Verification items for the finished model (mm, model axes). A direction names the side the tool comes from. Give positions to 0.01 mm unless a question says otherwise; leave off trailing zeros. Loops run counter-clockwise (first coordinate to the right, second up) from the corner with the lowest first, then second, coordinate; pieces in that order, holes last. Notation, with made-up numbers: M 50.5,24 L 86.5,24 A7 ccw 86.5,34 Z; hole C 56,4.25 d7. An arc over 180 degrees is marked long. Use a Markdown table: item, result.
from build123d import *

# Parameters (mm, degrees)
SKETCH1_R           = 25
BOSS_EXTRUDE1_DEPTH = 14
SKETCH2_R           = 11
CUT_EXTRUDE1_DEPTH  = 7
SKETCH5_W           = 7.5
SKETCH5_H           = 40
BOSS_EXTRUDE2_DEPTH = 80
FILLET1_R           = 10
SKETCH7_R           = 11
CUT_EXTRUDE3_DEPTH  = 24.5


with BuildPart() as part:
    # Sketch1 → Boss-Extrude1 (new body)
    with BuildSketch(Plane(origin=(0, 0, 0), x_dir=(1, 0, 0), z_dir=(0, 1, 0))):
        with Locations(Location((0, 0, 0), (0, 0, 90))):
            Circle(SKETCH1_R)
    extrude(amount=BOSS_EXTRUDE1_DEPTH)

    # Sketch2 → Cut-Extrude1 (cut)
    with BuildSketch(Plane.XZ):
        with Locations(Location((0, 0, 0), (0, 0, 270))):
            Circle(SKETCH2_R)
    extrude(amount=-CUT_EXTRUDE1_DEPTH, mode=Mode.SUBTRACT)

    # Sketch5 → Boss-Extrude2 (add)
    with BuildSketch(Plane(origin=(0, 14, 0), x_dir=(1, 0, 0), z_dir=(0, 1, 0))):
        with Locations((-8.85, 0)):
            Rectangle(SKETCH5_W, SKETCH5_H)
        with Locations((8.85, 0)):
            Rectangle(SKETCH5_W, SKETCH5_H)
    extrude(amount=BOSS_EXTRUDE2_DEPTH)

    # Fillet1
    fillet1_edges = [part.edges().sort_by_distance(p)[0] for p in [
        (-8.85, 94, 20),
        (-8.85, 94, -20),
        (8.85, 94, 20),
        (8.85, 94, -20),
    ]]
    fillet(fillet1_edges, radius=FILLET1_R)

    # Sketch7 → Cut-Extrude3 (cut)
    with BuildSketch(Plane.ZY.offset(12.6)):
        with Locations((0, 79)):
            Circle(SKETCH7_R)
    extrude(amount=-CUT_EXTRUDE3_DEPTH, mode=Mode.SUBTRACT)


solid = part.part
(1) Draft check along Z on faces 1 (the flat face through (11, 0, -5)), 2 (the cylindrical face through (8.9, 90.99, -17.15)), 3 (the flat face through (0, 7, 0)), 4 (the cylindrical face through (-8.8, 90.99, 17.15)). Enter one of: +Z half, -Z half, draft (parallel to the pull), parting line (faces both ways), or undercut.
Results below:
| item | result |
|---|---|
| face 1 | draft |
| face 2 | -Z half |
| face 3 | undercut |
| face 4 | +Z half |
(2) Material ranges on line 1 (X direction, y = 31.5, z = 17.5); line 2 (Y direction, x = 7.25, z = 0); line 3 (X direction, y = 4, z = 0), recorded low to high.
Results below:
| item | result |
|---|---|
| line 1 | -12.6 to -5.1, 5.1 to 12.6 |
| line 2 | 7 to 68, 90 to 94 |
| line 3 | -25 to -11, 11 to 25 |
(3) Set-up check for faces 5 (the flat face through (-5.1, 53, 0)), 6 (the flat face through (12.6, 53, 0)), 7 (the flat face through (9, 49, 20)), 8 (the cylindrical face through (8.452, 89.906, -1.432)), 9 (the flat face through (-9, 49, -20)): record each of +Z, -Z, +X, -X, +Y, -Y from which the full face is reachable in a straight line by a thin tool's end or side.
Results below:
| item | result |
|---|---|
| face 5 | +Z, -Z, +Y |
| face 6 | +Z, -Z, +X, +Y |
| face 7 | +Z, +X, -X, +Y |
| face 8 | -X |
| face 9 | -Z, +X, -X, +Y |
(4) Cross-section at A-A on y = 79. Record the cut outline in (x, z), then the cut area to 3 significant figures.
Results below:
| item | result |
|---|---|
| outline | M -12.6,-20 L -5.1,-20 L -5.1,-11 L -12.6,-11 Z; M -12.6,11 L -5.1,11 L -5.1,20 L -12.6,20 Z; M 5.1,-20 L 12.6,-20 L 12.6,20 L 5.1,20 L 5.1,11 L 11.9,11 L 11.9,-11 L 5.1,-11 Z |
| area | 285 mm^2 |
(5) Cross-section at C-C on z = 0. Record the cut outline in (x, y), then the cut area to 3 significant figures.
Results below:
| item | result |
|---|---|
| outline | M -25,0 L -11,0 L -11,7 L 11,7 L 11,0 L 25,0 L 25,14 L 12.6,14 L 12.6,94 L 5.1,94 L 5.1,90 L 11.9,90 L 11.9,68 L 5.1,68 L 5.1,14 L -5.1,14 L -5.1,68 L -12.6,68 L -12.6,14 L -25,14 Z; M -12.6,90 L -5.1,90 L -5.1,94 L -12.6,94 Z |
| area | 1,430 mm^2 |
(6) Cross-section at D-D on z = -5. Record the cut outline in (x, y), then the cut area to 3 significant figures.
Results below:
| item | result |
|---|---|
| outline | M -24.49,0 L -9.8,0 L -9.8,7 L 9.8,7 L 9.8,0 L 24.49,0 L 24.49,14 L 12.6,14 L 12.6,94 L 5.1,94 L 5.1,88.8 L 11.9,88.8 L 11.9,69.2 L 5.1,69.2 L 5.1,14 L -5.1,14 L -5.1,69.2 L -12.6,69.2 L -12.6,14 L -24.49,14 Z; M -12.6,88.8 L -5.1,88.8 L -5.1,94 L -12.6,94 Z |
| area | 1,470 mm^2 |
(7) Gauge pin test, flat ends, axial feed: P1, Ø8, axis at x = 10.5, y = 63, coming from the -Z side; P2, Ø1.5, axis at y = 75.5, z = -16, coming from the -X side; P3, Ø6, axis at y = 14, z = -13, coming from the -X side; P4, Ø13, axis at x = 0, z = 0, coming from the +Y side. Record the tip position at first contact, or that the pin passes through.
Results below:
| item | result |
|---|---|
| P1 | z = -20 |
| P2 | x = -12.6 |
| P3 | x = -22.91 |
| P4 | y = 94 |
(8) Cross-section at B-B on y = 40. Record the cut outline in (x, z), then the cut area to 3 significant figures.
Results below:
| item | result |
|---|---|
| outline | M -12.6,-20 L -5.1,-20 L -5.1,20 L -12.6,20 Z; M 5.1,-20 L 12.6,-20 L 12.6,20 L 5.1,20 Z |
| area | 600 mm^2 |
